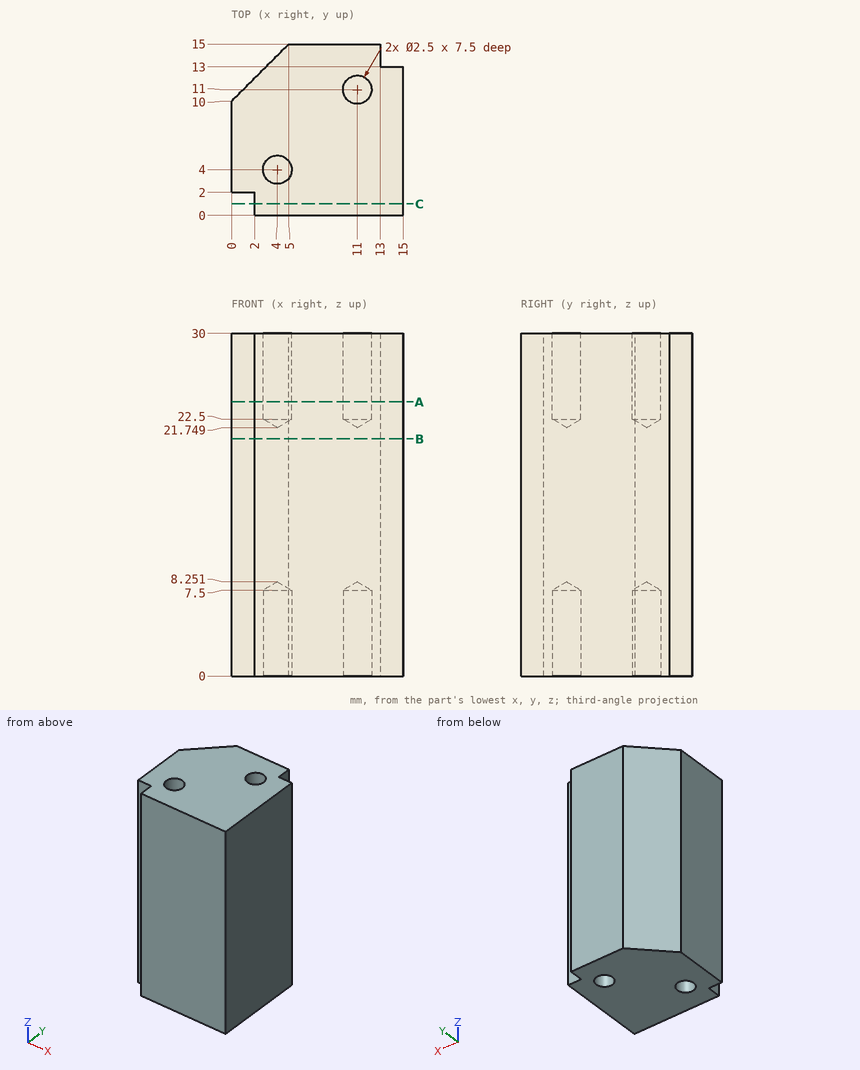
The drawing under review shows one solid part. Ordinate dimensions are in mm from its lowest x, y, z. Coordinates: 2 decimals unless noted, no trailing zeros. Order: outer loops, then holes, each group sorted by start corner. A loop starts at its lowest first (then second) coordinate and runs counter-clockwise, first axis right, second up. Notation, with made-up numbers: (54.25, 2) -> (64.25, 2) arc R8 cw to (64.25, 6) -> close; hole circle Ø6 at (14.25, 58.5). An arc over 180 degrees is marked (long way). Answer as CSV lines item,"result".
Q1. Wall thickness on line 1 along Y through (x, z) = (11, 27.75); line 2 along X through (y, z) = (4, 2); line 3 along Y through (x, z) = (3.5, 24.5): over which ranges is each line inside the solid? List them lowest first. Write a range as [from, to].
Model answer:
line 1,"y = [0, 9.75], [12.25, 15]"
line 2,"x = [0, 2.75], [5.25, 15]"
line 3,"y = [0, 2.85], [5.15, 13.5]"
Q2. Clearance check with flat-ended pins moving along their axes: pin 1 Ø3 at (x, y) = (4, 4) entering from -Z; pin 2 Ø1.5 at (x, y) = (11, 11) entering from -Z; pin 3 Ø0.6 at (x, z) = (14, 13) entering from +Y; pin 4 Ø1 at (x, z) = (1, 12) entering from -Y. State where each tip first meets the part, or that it passes through.
Model answer:
pin 1,"stops at z = 0"
pin 2,"stops at z = 7.8"
pin 3,"stops at y = 13"
pin 4,"stops at y = 2"
Q3. We need section C-C (y = 1). State the section outline as (x, z) points, plus the area to 3 significant figures.
Model answer:
outline,"(2, 0) -> (15, 0) -> (15, 30) -> (2, 30) -> close"
area,"390 mm2"
Q4. We need section B-B (z = 20.75). State the section outline as (x, y) points.
Model answer:
outline,"(0, 2) -> (2, 2) -> (2, 0) -> (15, 0) -> (15, 13) -> (13, 13) -> (13, 15) -> (5, 15) -> (0, 10) -> close"
Q5. We need section A-A (z = 24). State the section outline as (x, y) points.
Model answer:
outline,"(0, 2) -> (2, 2) -> (2, 0) -> (15, 0) -> (15, 13) -> (13, 13) -> (13, 15) -> (5, 15) -> (0, 10) -> close; hole circle Ø2.5 at (4, 4); hole circle Ø2.5 at (11, 11)"
